Answer from the drawing. Dimensions are ordinates in mm from the lowest x, y and z of the part. A direction names the side the tool comes from. Round coordinates to 2 decimals unless told otherwise and drop trailing zeros. Loops run counter-clockwise (first coordinate to the right, second up) from the corner with the lowest first, then second, coordinate; pieces in that order, holes last.
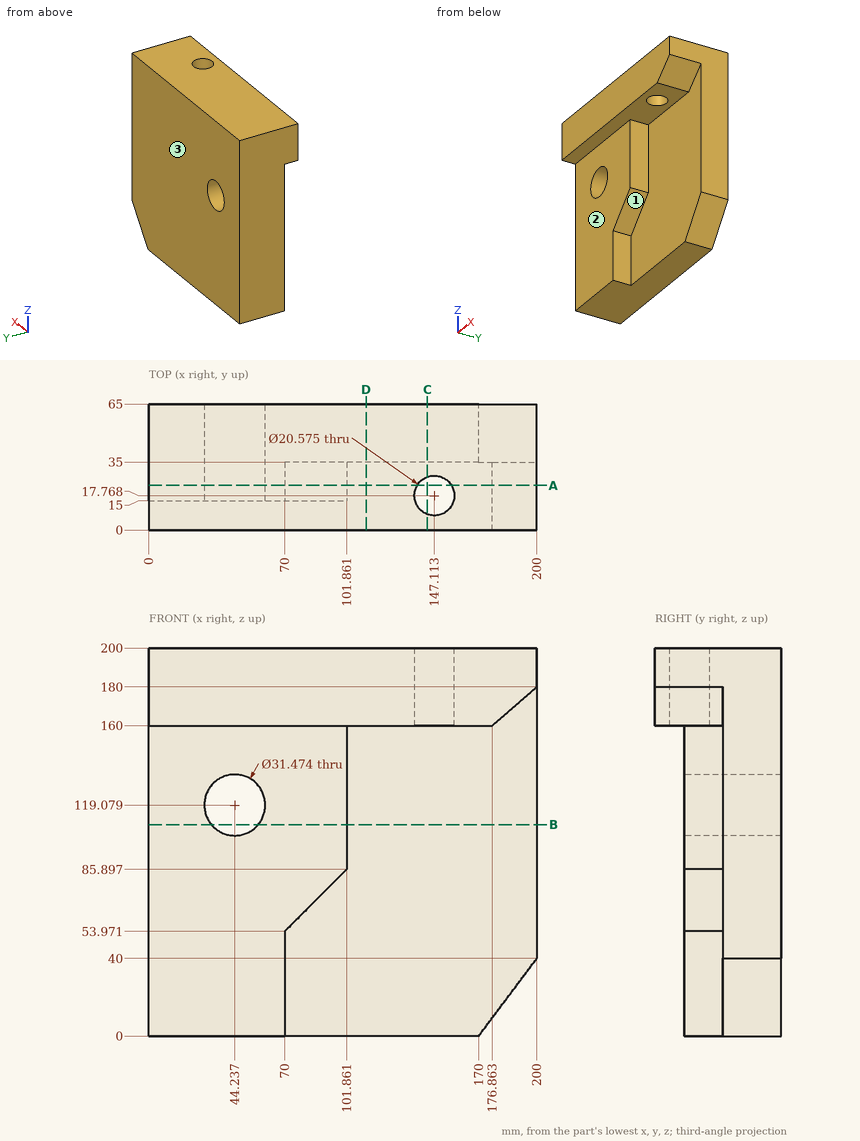
1. Find section D-D (x = 112). Write down the section's boundary in (y, z).
Answer key:
outline: (0, 160) - (35, 160) - (35, 0) - (65, 0) - (65, 200) - (0, 200) - close
2. Given pin 1 (10 mm diameter, centred on x = 124.5, z = 122, fed in from -Y); pin 2 (5 mm diameter, centred on y = 40, z = 169, fed in from -X); pin 3 (10 mm diameter, centred on x = 24, z = 38.5, fed in from -Y); pin 4 (22 mm diameter, centred on y = 22, z = 139, fed in from +X), each flat-ended and moving along its own axis, determine where each tip first touches the part or whether it passes through.
Answer key:
pin 1: stops at y = 35
pin 2: stops at x = 0
pin 3: stops at y = 15
pin 4: stops at x = 101.86
3. Find section C-C (x = 143.5). Write down the section's boundary in (y, z) (1 decimal).
Answer key:
outline: (0, 160) - (8.1, 160) - (8.1, 200) - (0, 200) - close; (27.4, 160) - (35, 160) - (35, 0) - (65, 0) - (65, 200) - (27.4, 200) - close
4. Find section A-A (y = 23). Write down the section's boundary in (x, z) (1 decimal).
Answer key:
outline: (0, 0) - (70, 0) - (70, 54) - (101.9, 85.9) - (101.9, 160) - (138.3, 160) - (138.3, 200) - (0, 200) - close; (156, 160) - (176.9, 160) - (200, 180) - (200, 200) - (156, 200) - close; hole circle Ø31.5 at (44.2, 119.1)
5. Find section B-B (z = 109). Write down the section's boundary in (x, y).
Answer key:
outline: (0, 15) - (32.15, 15) - (32.15, 65) - (0, 65) - close; (56.32, 15) - (101.86, 15) - (101.86, 35) - (200, 35) - (200, 65) - (56.32, 65) - close
6. Consider probe 1 along X at (y, z) = (44.5, 120); probe 2 along Y at (x, z) = (9.5, 148.5); probe 3 along Y at (x, z) = (181, 69). Determine where each line is inside the solid, lowest interval first.
Answer key:
probe 1: x = 0 to 28.53, 59.95 to 200
probe 2: y = 15 to 65
probe 3: y = 35 to 65
7. Which of the six approach directions +Z, -Z, +X, -X, +Y, -Y give full straight-line access (tool end or side, diameter ignored) to the marked faces 1, 2 and 3?
Answer key:
face 1: -Z, +X, -Y
face 2: -Z, +X, -X, -Y
face 3: +Z, -Z, +X, -X, +Y
